Source: CAD feature listing. Evaluate the final solid. Frame: model axes, mm. Face numbers are marked on the shaded views. A direction names the side the tool comes from. Give positions to 0.01 mm unless a question says otherwise; leave off trailing zeros. Order: outer loops, then holes, each group sorted by start corner. A loop starts at its lowest first (then second) coordinate and runs counter-clockwise, first axis right, second up. Notation, with made-up numbers: M 83,57 L 129,57 A11 ccw 129,77 Z; hole C 59,-37.5 d8. An arc over 180 degrees is marked long. Use CSV: the item, a comma, the result in double quotes. Start each with the question number.
1. Reachability of the marked faces 1 and 2 from +Z, -Z, +X, -X, +Y, -Y: full face, straight path, thin tool, end or side. Return the list, or none.
2. Section query A-A, the plane x = 12.5. Return the cut outline in (y, z).
3. Section query B-B, the plane z = -15. Return the cut outline in (x, y).
4. Line query: line 1 along Y through (x, z) = (3, -23.25); line 2 along Z through (x, y) = (4.5, 2.25). Output: solid intervals per line, ascending. Write a range as [from, to].
5. Section query C-C, the plane y = 13.5. Return the cut outline in (x, z), plus the area to 3 significant figures.
6. Pin query (flat end, axial travel): P1, Ø1, axis at x = 3.5, y = 15.5, coming from the -Z side; P2, Ø1.5, axis at x = 17.5, z = -5, coming from the +Y side; P3, Ø10, axis at y = 7, z = -22, coming from the +X side. Return the tip coordinate at first contact, or that it passes through.
from build123d import *

# Parameters (mm, degrees)
SKETCH1_W           = 25.4
SKETCH1_H           = 25.4
BOSS_EXTRUDE1_DEPTH = 0.79375
SKETCH2_W           = 0.79375
SKETCH2_H           = 25.4
BOSS_EXTRUDE2_DEPTH = 25.4


with BuildPart() as part:
    # Sketch1 → Boss-Extrude1 (new body)
    with BuildSketch(Plane(origin=(0, 0, 0), x_dir=(1, 0, 0), z_dir=(0, 1, 0))):
        with Locations((12.7, 12.7)):
            Rectangle(SKETCH1_W, SKETCH1_H)
    extrude(amount=BOSS_EXTRUDE1_DEPTH)

    # Sketch2 → Boss-Extrude2 (add)
    with BuildSketch(Plane(origin=(25.4, 0, 0), x_dir=(0, 0, -1), z_dir=(1, 0, 0))):
        with Locations((0.396875, 12.7)):
            Rectangle(SKETCH2_W, SKETCH2_H)
    extrude(amount=-BOSS_EXTRUDE2_DEPTH)


solid = part.part
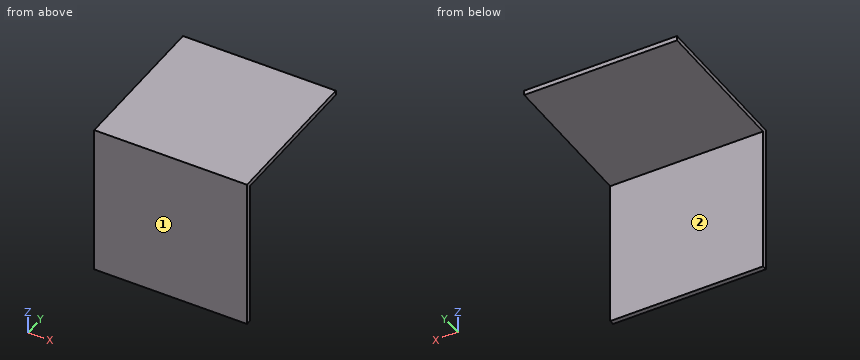
Result set:
1,face 1,"+Z, -Z, +X, -X, -Y"
1,face 2,"-Z, +X, -X, +Y"
2,outline,"M 0,-25.4 L 0.79,-25.4 L 0.79,-0.79 L 25.4,-0.79 L 25.4,0 L 0,0 Z"
3,outline,"M 0,0 L 25.4,0 L 25.4,0.79 L 0,0.79 Z"
4,line 1,"[0, 0.79]"
4,line 2,"[-0.79, 0]"
5,outline,"M 0,-0.79 L 25.4,-0.79 L 25.4,0 L 0,0 Z"
5,area,"20.2 mm2"
6,P1,"z = -0.79"
6,P2,"y = 0.79"
6,P3,"through"
